The figure shows three views and two pictorial views of one solid part (mm, origin at its lowest corner). Answer the questions. Round coordinates to 2 decimals unless told otherwise and drop trailing zeros. Write each loop counter-clockwise with the first axis right and the second up, starting at its lowest first coordinate (ties: lowest second). Pieces come first, ordered by that corner, then holes. Notation, with made-up numbers: M 49,19.5 L 67,19.5 A27 cw 67,53.5 Z; hole C 85.25,67 d6. An arc over 180 degrees is marked long. One line per item, written item: value. Start each with the question number.
Q1. Find section C-C (x = 43.5). Write down the section's boundary in (y, z), and give its area (3 significant figures).
Q2. Find section A-A (y = 3.9). Write down the section's boundary in (x, z).
Q3. Given pin 1 Ø1.5 at (x, y) = (19, 3) entering from -Z; pin 2 Ø10 at (x, z) = (30.5, 41.5) entering from +Y, each flat-ended and moving along its own axis, determine where each tip first touches the part or whether it passes through.
Q4. Consider probe 1 along Z at (x, y) = (39.5, 0.3); probe 2 along Z at (x, y) = (43.5, 4.5); probe 3 along X at (y, z) = (1.95, 50). Determine where each line is inside the solid, lowest interval first.
Q5. Find section B-B (z = 54). Write down the section's boundary in (x, y).
Q6. Find section D-D (x = 16.5). Write down the section's boundary in (y, z), and give its area (4 significant figures).
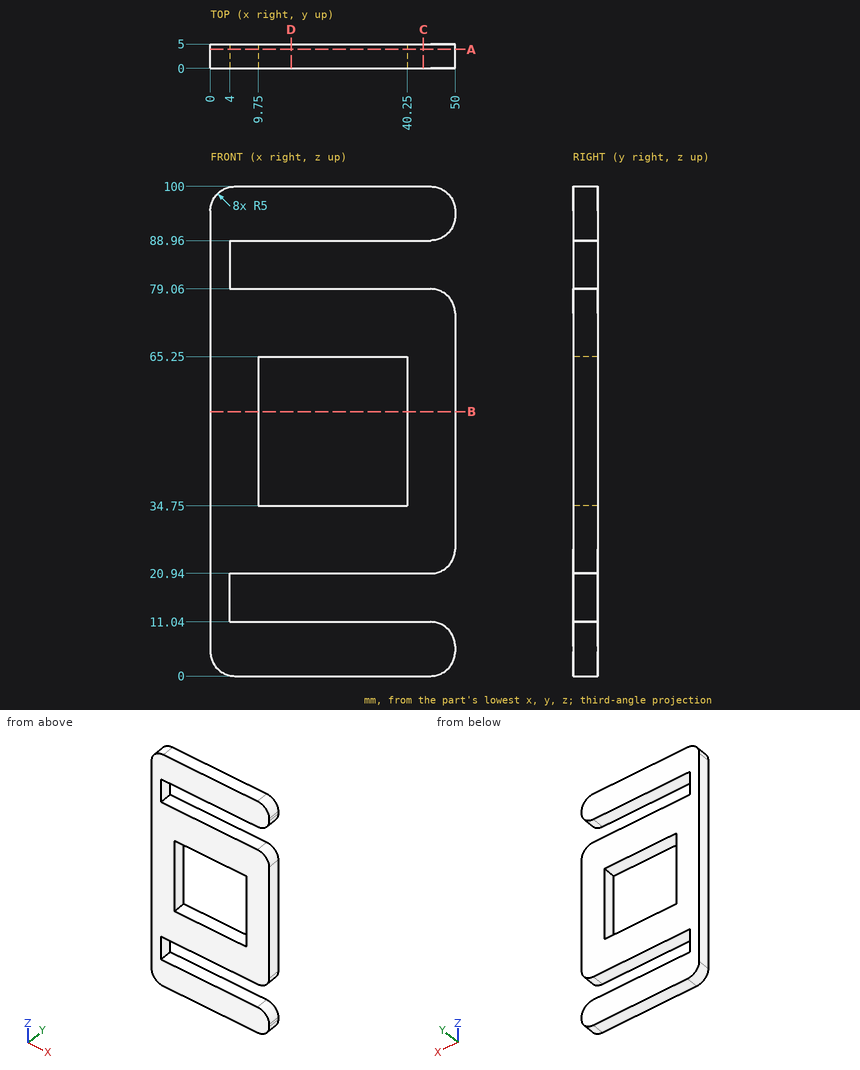
The answers:
1. outline: M 0,0 L 5,0 L 5,11.04 L 0,11.04 Z; M 0,20.94 L 5,20.94 L 5,79.06 L 0,79.06 Z; M 0,88.96 L 5,88.96 L 5,100 L 0,100 Z
1. area: 401 mm2
2. outline: M 0,5 A5 ccw 5,0 L 45,0 A5 ccw 50,5 L 50,6.04 A5 ccw 45,11.04 L 4,11.04 L 4,20.94 L 45,20.94 A5 ccw 50,25.94 L 50,74.06 A5 ccw 45,79.06 L 4,79.06 L 4,88.96 L 45,88.96 A5 ccw 50,93.96 L 50,95 A5 ccw 45,100 L 5,100 A5 ccw 0,95 Z; hole M 9.75,34.75 L 40.25,34.75 L 40.25,65.25 L 9.75,65.25 Z
3. pin 1: z = 0
3. pin 2: through
4. probe 1: 0 to 11.04, 20.94 to 34.75, 65.25 to 79.06, 88.96 to 100
4. probe 2: 0 to 11.04, 20.94 to 79.06, 88.96 to 100
4. probe 3: 0 to 9.75, 40.25 to 50
5. outline: M 0,0 L 9.75,0 L 9.75,5 L 0,5 Z; M 40.25,0 L 50,0 L 50,5 L 40.25,5 Z
6. outline: M 0,0 L 5,0 L 5,11.04 L 0,11.04 Z; M 0,20.94 L 5,20.94 L 5,34.75 L 0,34.75 Z; M 0,65.25 L 5,65.25 L 5,79.06 L 0,79.06 Z; M 0,88.96 L 5,88.96 L 5,100 L 0,100 Z
6. area: 248.5 mm2
